from build123d import *

# Parameters (mm, degrees)
SKETCH1_W                                        = 22
SKETCH1_H                                        = 28
BOSS_EXTRUDE1_DEPTH                              = 9.5
SKETCH2_W                                        = 17.45
SKETCH2_H                                        = 1.5
CUT_EXTRUDE1_DEPTH                               = 23
CUT_EXTRUDE2_DEPTH                               = 4.85
SKETCH4_W                                        = 4.55
SKETCH4_H                                        = 1.5
CUT_EXTRUDE3_DEPTH                               = 23
CBORE_FOR_M4_HEX_HEAD_MACHINE_SCREW1_D           = 4.3
CBORE_FOR_M4_HEX_HEAD_MACHINE_SCREW1_DEPTH       = 9.5
CBORE_FOR_M4_HEX_HEAD_MACHINE_SCREW1_CBORE_D     = 8.5
CBORE_FOR_M4_HEX_HEAD_MACHINE_SCREW1_CBORE_DEPTH = 5
FILLET1_R                                        = 1
FILLET2_R                                        = 0.5
FILLET3_R                                        = 2


with BuildPart() as part:
    # Sketch1 → Boss-Extrude1 (new body)
    with BuildSketch(Plane(origin=(0, 8, 0), x_dir=(1, 0, 0), z_dir=(0, 1, 0))):
        Rectangle(SKETCH1_W, SKETCH1_H)
    extrude(amount=-BOSS_EXTRUDE1_DEPTH)

    # Sketch2 → Cut-Extrude1 (cut, through all)
    with BuildSketch(Plane(origin=(11, 0, 0), x_dir=(0, 0, -1), z_dir=(1, 0, 0))):
        with Locations((-5.275, -0.75)):
            Rectangle(SKETCH2_W, SKETCH2_H)
    extrude(amount=-CUT_EXTRUDE1_DEPTH, mode=Mode.SUBTRACT)

    # Sketch3 → Cut-Extrude2 (cut)
    with BuildSketch(Plane(origin=(0, 8, 0), x_dir=(-1, 0, 0), z_dir=(0, 1, 0))):
        with BuildLine():
            Line((11, 7.358592124), (11, 14))
            Line((11, 14), (-11, 14))
            Line((-11, 14), (-11, -3.718814308))
            ThreePointArc((-11, -3.718814308), (0.2873816, 1.249142024), (11, 7.358592124))
        make_face()
    extrude(amount=-CUT_EXTRUDE2_DEPTH, mode=Mode.SUBTRACT)

    # Sketch4 → Cut-Extrude3 (cut, through all)
    with BuildSketch(Plane(origin=(11, 0, 0), x_dir=(0, 0, -1), z_dir=(1, 0, 0))):
        with Locations((11.725, -0.75)):
            Rectangle(SKETCH4_W, SKETCH4_H)
    extrude(amount=-CUT_EXTRUDE3_DEPTH, mode=Mode.SUBTRACT)

    # CBORE for M4 Hex Head Machine Screw1
    with Locations(Plane(origin=(0, 8, 0), x_dir=(1, 0, 0), z_dir=(0, 1, 0))):
        with Locations((0, 6.45)):
            CounterBoreHole(CBORE_FOR_M4_HEX_HEAD_MACHINE_SCREW1_D / 2, CBORE_FOR_M4_HEX_HEAD_MACHINE_SCREW1_CBORE_D / 2, CBORE_FOR_M4_HEX_HEAD_MACHINE_SCREW1_CBORE_DEPTH, depth=CBORE_FOR_M4_HEX_HEAD_MACHINE_SCREW1_DEPTH)

    # Fillet1
    fillet1_edges = [part.edges().sort_by_distance(p)[0] for p in [
        (-11, -0.75, -3.45),
        (11, -0.75, -3.45),
        (-11, -0.75, -9.45),
        (11, -0.75, -9.45),
    ]]
    fillet(fillet1_edges, radius=FILLET1_R)

    # Fillet2
    fillet2_edges = [part.edges().sort_by_distance(p)[0] for p in [
        (0, -1.5, -3.45),
        (11, -1.5, -6.45),
        (-11, -1.5, -6.45),
        (0, -1.5, -9.45),
        (-10.707106781, -1.5, -9.157106781),
        (10.707106781, -1.5, -9.157106781),
        (-10.707106781, -1.5, -3.742893219),
        (10.707106781, -1.5, -3.742893219),
    ]]
    fillet(fillet2_edges, radius=FILLET2_R)

    # Fillet3
    fillet3_edges = [part.edges().sort_by_distance(p)[0] for p in [
        (11, 1.575, 14),
        (-11, 1.575, 14),
        (11, 4, -14),
        (-11, 4, -14),
    ]]
    fillet(fillet3_edges, radius=FILLET3_R)


solid = part.part
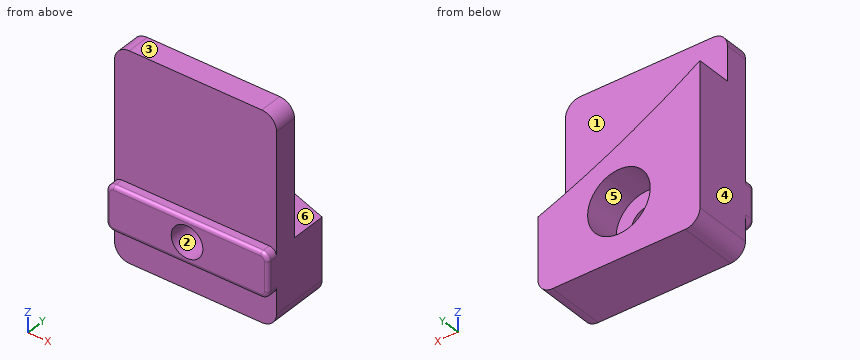
Design review of the part built by this model. Coordinates are the model's own, in mm. Face numbers are marked on the shaded views. A direction names the side the tool comes from. Round coordinates to 2 decimals unless told otherwise and drop trailing zeros. Order: outer loops, then holes, each group sorted by start corner. A loop starts at its lowest first (then second) coordinate and runs counter-clockwise, first axis right, second up.
1) Consider section D-D (y = -0.5). State the section outline as (x, z) points.
The answers:
outline: (-11, -8.45) arc R1 ccw to (-10, -9.45) - (10, -9.45) arc R1 ccw to (11, -8.45) - (11, -4.45) arc R1 ccw to (10, -3.45) - (-10, -3.45) arc R1 ccw to (-11, -4.45) - close; hole circle Ø4.3 at (0, -6.45)
2) Consider section B-B (z = -6.45). State the section outline as (x, y) points.
The answers:
outline: (-11, -1) arc R0.5 ccw to (-10.5, -1.5) - (-2.15, -1.5) - (-2.15, 3) - (-4.25, 3) - (-4.25, 8) - (-11, 8) - close; (2.15, -1.5) - (10.5, -1.5) arc R0.5 ccw to (11, -1) - (11, 8) - (4.25, 8) - (4.25, 3) - (2.15, 3) - close
3) Consider section C-C (x = 0). State the section outline as (y, z) points, plus the area to 3 significant figures.
The answers:
outline: (-1.5, -8.95) arc R0.5 ccw to (-1, -9.45) - (0, -9.45) - (0, -14) - (8, -14) - (8, -10.7) - (3, -10.7) - (3, -8.6) - (-1.5, -8.6) - close; (-1.5, -4.3) - (3, -4.3) - (3, -2.2) - (8, -2.2) - (8, 1.1) - (3.15, 1.1) - (3.15, 14) - (0, 14) - (0, -3.45) - (-1, -3.45) arc R0.5 ccw to (-1.5, -3.95) - close
area: 109 mm2
4) Machinability: for the marked faces 4, 5 and 6, which of the approach directions +Z, -Z, +X, -X, +Y, -Y give a long, thin tool a straight path to every point of the face, cutting with its end or side? Answer none if there is none.
The answers:
face 4: +Z, -Z, -X, +Y, -Y
face 5: +Y
face 6: +Z, +X, +Y
5) Consider section A-A (y = 4.5). State the section outline as (x, z) points, plus the area to 3 significant figures.
The answers:
outline: (-11, -12) arc R2 ccw to (-9, -14) - (9, -14) arc R2 ccw to (11, -12) - (11, -3.72) arc R119 cw to (-11, 7.36) - close; hole circle Ø8.5 at (0, -6.45)
area: 279 mm2
6) For L1, parallel to Y at x = 8.5, z = 6.75; L2, parallel to Z at x = 0, y = 1.45; L3, parallel to Y at x = -9.75, z = 0.75, list the stretches that pass through material, from the lowest coordinate up.
The answers:
L1: y = 0 to 3.15
L2: z = -14 to -8.6, -4.3 to 14
L3: y = 0 to 8
7) Clearance check with flat-ended pins moving along their axes: pin 1 Ø2 at (x, y) = (7, 6) entering from +Z; pin 2 Ø4 at (x, z) = (0, -6.45) entering from +Y (3 decimals); pin 3 Ø0.5 at (x, y) = (0, -0.5) entering from -Z; pin 4 Ø4 at (x, z) = (1.5, -6) entering from +Y. State where each tip first meets the part, or that it passes through.
The answers:
pin 1: stops at z = -1.69
pin 2: passes through
pin 3: stops at z = -9.45
pin 4: stops at y = 3
8) Draft analysis for pull direction Z (two halves, no side actions). For the marked faces 1, 2 and 3, state which applies: released by +Z, released by -Z, zero draft, split by the parting line, or undercut.
The answers:
face 1: zero draft
face 2: undercut
face 3: released by +Z
